For this review, take the finished solid that the model builds, in its own axes (mm). A direction names the side the tool comes from. Give positions to 0.01 mm unless a question says otherwise; leave off trailing zeros. Loops run counter-clockwise (first coordinate to the right, second up) from the corner with the lowest first, then second, coordinate; pieces in that order, holes last. Notation, with made-up numbers: (81.25, 65) - (98.25, 65) arc R22 ccw to (98.25, 83) - close; hole circle Ø7 at (12, 24.5). An arc over 180 degrees is marked (long way). Answer in a Markdown table with one row per item.
```python
from build123d import *

# Parameters (mm, degrees)
SKETCH1_R           = 123.75
BOSS_EXTRUDE1_DEPTH = 8
SKETCH2_R           = 1.905
CUT_EXTRUDE2_DEPTH  = 9
CIRPATTERN1_COUNT   = 4
SKETCH3_R           = 4.5
CUT_EXTRUDE3_DEPTH  = 9
SKETCH4_R           = 3.81
CUT_EXTRUDE4_DEPTH  = 2.54
CIRPATTERN2_COUNT   = 4
SKETCH5_W           = 10
SKETCH5_H           = 30
CUT_EXTRUDE5_DEPTH  = 9


with BuildPart() as part:
    # Sketch1 → Boss-Extrude1 (new body)
    with BuildSketch(Plane(origin=(0, 0, 0), x_dir=(1, 0, 0), z_dir=(0, 1, 0))):
        Circle(SKETCH1_R)
    extrude(amount=BOSS_EXTRUDE1_DEPTH)

    # Sketch2 → Cut-Extrude2 (cut, through all)
    with BuildSketch(Plane(origin=(0, 8, 0), x_dir=(1, 0, 0), z_dir=(0, 1, 0))):
        with Locations((0, 9.779)):
            Circle(SKETCH2_R)
    cut_extrude2 = extrude(amount=-CUT_EXTRUDE2_DEPTH, mode=Mode.SUBTRACT)

    # CirPattern1: Cut-Extrude2 ×4 about axis
    cirpattern1_axis = Axis((0, 0, 0), (0, 1, 0))
    for i in range(1, CIRPATTERN1_COUNT):
        add(cut_extrude2.rotate(cirpattern1_axis, i * 360 / CIRPATTERN1_COUNT), mode=Mode.SUBTRACT)

    # Sketch3 → Cut-Extrude3 (cut, through all)
    with BuildSketch(Plane(origin=(0, 8, 0), x_dir=(1, 0, 0), z_dir=(0, 1, 0))):
        Circle(SKETCH3_R)
    extrude(amount=-CUT_EXTRUDE3_DEPTH, mode=Mode.SUBTRACT)

    # Sketch4 → Cut-Extrude4 (cut)
    with BuildSketch(Plane(origin=(0, 8, 0), x_dir=(1, 0, 0), z_dir=(0, 1, 0))):
        with Locations((0, 9.779)):
            Circle(SKETCH4_R)
    cut_extrude4 = extrude(amount=-CUT_EXTRUDE4_DEPTH, mode=Mode.SUBTRACT)

    # CirPattern2: Cut-Extrude4 ×4 about axis
    cirpattern2_axis = Axis((0, 0, 0), (0, 1, 0))
    for i in range(1, CIRPATTERN2_COUNT):
        add(cut_extrude4.rotate(cirpattern2_axis, i * 360 / CIRPATTERN2_COUNT), mode=Mode.SUBTRACT)

    # Sketch5 → Cut-Extrude5 (cut, through all)
    with BuildSketch(Plane(origin=(0, 8, 0), x_dir=(1, 0, 0), z_dir=(0, 1, 0))):
        with Locations((75, 0)):
            Rectangle(SKETCH5_W, SKETCH5_H)
        with Locations((-75, 0)):
            Rectangle(SKETCH5_W, SKETCH5_H)
    extrude(amount=-CUT_EXTRUDE5_DEPTH, mode=Mode.SUBTRACT)


solid = part.part
```
1. For faces 1 (the face through (-12, 5.46, -1)), 2 (the face through (75, 4, -15)), list the 3-axis set-ups (+Z, -Z, +X, -X, +Y, -Y) from which the entire face can be reached by the end or side of a thin tool; tool diameter is ignored.
Values:
| item | result |
|---|---|
| face 1 | +Y |
| face 2 | +Y, -Y |
2. Clearance check with flat-ended pins moving along their axes: pin 1 (6 mm diameter, centred on x = 0.5, z = 10, fed in from +Y); pin 2 (1.5 mm diameter, centred on x = -36, z = 17.5, fed in from -Y); pin 3 (3 mm diameter, centred on y = 4.5, z = -90, fed in from -X); pin 4 (4 mm diameter, centred on x = -76, y = 4.5, fed in from +Z). State where each tip first meets the part, or that it passes through.
Values:
| item | result |
|---|---|
| pin 1 | stops at y = 5.46 |
| pin 2 | stops at y = 0 |
| pin 3 | stops at x = -86.5 |
| pin 4 | stops at z = 99.19 |
3. We need section A-A, the plane y = 3.25. Give the boundary of the cut face in (x, z) (3 decimals).
Values:
| item | result |
|---|---|
| outline | circle Ø247.5 at (0, 0); hole (-80, -15) - (-70, -15) - (-70, 15) - (-80, 15) - close; hole circle Ø3.81 at (-9.779, 0); hole circle Ø9 at (0, 0); hole circle Ø3.81 at (0, -9.779); hole circle Ø3.81 at (0, 9.779); hole circle Ø3.81 at (9.779, 0); hole (70, -15) - (80, -15) - (80, 15) - (70, 15) - close |
4. Wall thickness on line 1 (Z direction, x = 0, y = 5); line 2 (X direction, y = 6.2, z = 0); line 3 (X direction, y = 1.4, z = 0): over which ranges is each line inside the solid? List them lowest first. Write a range as [from, to].
Values:
| item | result |
|---|---|
| line 1 | z = [-123.75, -11.68], [-7.87, -4.5], [4.5, 7.87], [11.68, 123.75] |
| line 2 | x = [-123.75, -80], [-70, -13.59], [-5.97, -4.5], [4.5, 5.97], [13.59, 70], [80, 123.75] |
| line 3 | x = [-123.75, -80], [-70, -11.68], [-7.87, -4.5], [4.5, 7.87], [11.68, 70], [80, 123.75] |
5. We need section D-D, the plane x = 26. Give the boundary of the cut face in (y, z).
Values:
| item | result |
|---|---|
| outline | (0, -120.99) - (8, -120.99) - (8, 120.99) - (0, 120.99) - close |
6. We need section B-B, the plane x = 76.5. Give the boundary of the cut face in (y, z).
Values:
| item | result |
|---|---|
| outline | (0, -97.27) - (8, -97.27) - (8, -15) - (0, -15) - close; (0, 15) - (8, 15) - (8, 97.27) - (0, 97.27) - close |
7. We need section C-C, the plane z = -74.5. Give the boundary of the cut face in (x, y), and give its area (3 significant figures).
Values:
| item | result |
|---|---|
| outline | (-98.81, 0) - (98.81, 0) - (98.81, 8) - (-98.81, 8) - close |
| area | 1,580 mm^2 |
8. Mouldability with a two-part tool opening along X and no side actions: class faces 3 (the face through (-2, 0, 26)), 4 (the face through (-75, 4, -15)), 5 (the face through (-16.1, 3.9, -122.7)), 6 (the face through (-0.496, 6.748, -13.557)) as released by +X, released by -X, zero draft, split by the parting line, or undercut.
Values:
| item | result |
|---|---|
| face 3 | zero draft |
| face 4 | undercut |
| face 5 | split by the parting line |
| face 6 | undercut |
